Check sheet for the drawn part. Datum: minimum x, y, z corner. Units: mm. Give positions to 0.01 mm unless a question says otherwise; leave off trailing zeros. Write each loop counter-clockwise with the first axis right and the second up, starting at its lowest first coordinate (ties: lowest second). Pieces come first, ordered by that corner, then holes. Notation, with made-up numbers: M 8.25,33 L 50.25,33 A35 ccw 50.25,70 Z; hole C 85.5,38.25 d6. An arc over 180 degrees is marked long. Write item = value, one per line. Start each with the question number.
1) Draft check along Y on the marked faces 1, 2, 3 and 4. Enter one of: pulls with the +Y half, pulls with the -Y half, needs draft (parallel to the pull), parting line crosses it, or undercut.
2) Sectioned sample at B-B, the plane y = 6.5. Record the cut outline in (x, z).
3) Sectioned sample at D-D, the plane y = 23.75. Record the cut outline in (x, z).
4) Scan lines: L1, parallel to Y at x = 5, z = 1.7; L2, parallel to X at y = 20, z = 2.7; L3, parallel to X at y = 7, z = 3.5. Record each from-to range of solid material in increasing order.
5) Sectioned sample at A-A, the plane z = 3.55. Record the cut outline in (x, y), then the cut area to 3 significant figures.
6) Sectioned sample at C-C, the plane y = 20.75. Record the cut outline in (x, z).
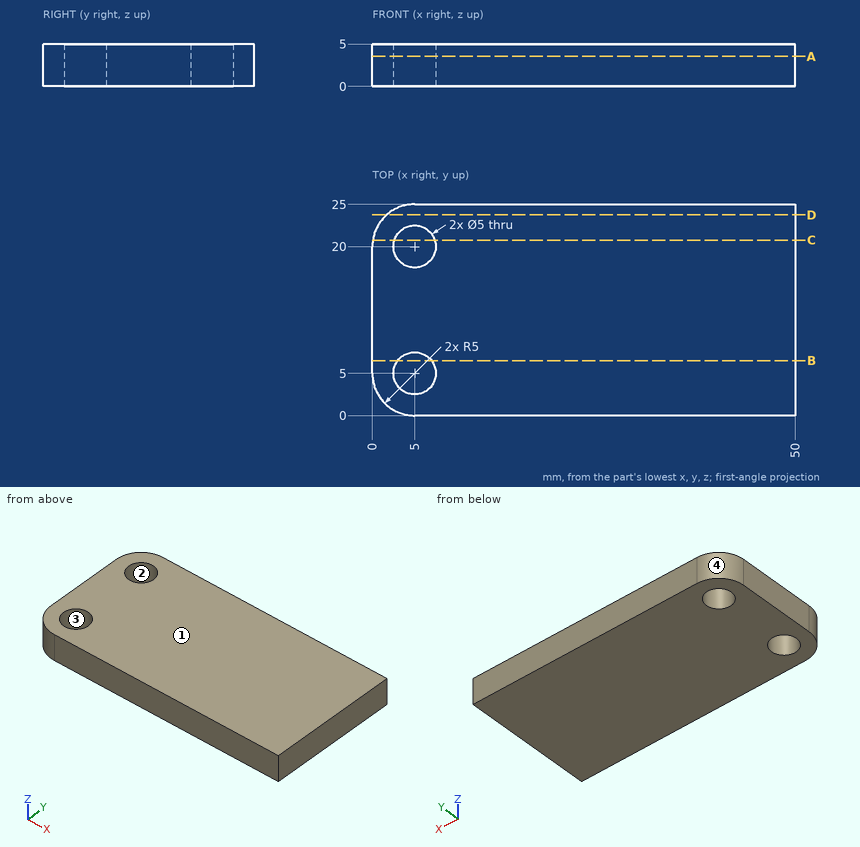
Data:
q1.face_1 = needs draft
q1.face_2 = undercut
q1.face_3 = undercut
q1.face_4 = pulls with the +Y half
q2.outline = M 0,0 L 3,0 L 3,5 L 0,5 Z; M 7,0 L 50,0 L 50,5 L 7,5 Z
q3.outline = M 1.69,0 L 50,0 L 50,5 L 1.69,5 Z
q4.L1 = 0 to 2.5, 7.5 to 17.5, 22.5 to 25
q4.L2 = 0 to 2.5, 7.5 to 50
q4.L3 = 0 to 3.5, 6.5 to 50
q5.outline = M 0,5 A5 ccw 5,0 L 50,0 L 50,25 L 5,25 A5 ccw 0,20 Z; hole C 5,5 d5; hole C 5,20 d5
q5.area = 1,200 mm2
q6.outline = M 0.06,0 L 2.62,0 L 2.62,5 L 0.06,5 Z; M 7.38,0 L 50,0 L 50,5 L 7.38,5 Z
